Verification items for the finished model (mm, model axes). A direction names the side the tool comes from. Coordinates: 2 decimals unless noted, no trailing zeros. Order: outer loops, then holes, each group sorted by start corner. A loop starts at its lowest first (then second) coordinate and runs counter-clockwise, first axis right, second up. Notation, with made-up numbers: M 33,-2.75 L 77,-2.75 A20 ccw 77,1.25 Z; hole C -16.75,84.5 d1. An arc over 180 degrees is marked long. Return JSON: item names as keys, results as strings.
```python
from build123d import *

# Parameters (mm, degrees)
ESQUISSE1_W             = 170
ESQUISSE1_H             = 80
BOSS_EXTRU_1_DEPTH      = 3
ESQUISSE3_W             = 28
ESQUISSE3_H             = 3
ESQUISSE3_W_2           = 22
BOSS_EXTRU_2_DEPTH      = 3
ESQUISSE4_W             = 3
ESQUISSE4_H             = 19
ESQUISSE4_H_2           = 18
ESQUISSE4_H_3           = 19.233956883
BOSS_EXTRU_3_DEPTH      = 3
ESQUISSE5_W             = 3.071340823
ESQUISSE5_H             = 0.315544452
ENL_V_MAT_EXTRU_1_DEPTH = 3


with BuildPart() as part:
    # Esquisse1 → Boss.-Extru.1 (new body)
    with BuildSketch(Plane.XY):
        with Locations((40.41093995, 17.47440273)):
            Rectangle(ESQUISSE1_W, ESQUISSE1_H)
    extrude(amount=BOSS_EXTRU_1_DEPTH)

    # Esquisse3 → Boss.-Extru.2 (add)
    with BuildSketch(Plane(origin=(0, 0, 0), x_dir=(-1, 0, 0), z_dir=(0, 0, -1))):
        with Locations((-0.41093995, 58.97440273)):
            Rectangle(ESQUISSE3_W, ESQUISSE3_H)
        with Locations((-60.41093995, 58.97440273)):
            Rectangle(ESQUISSE3_W, ESQUISSE3_H)
        with Locations((-117.41093995, 58.97440273)):
            Rectangle(ESQUISSE3_W_2, ESQUISSE3_H)
        with Locations((-117.41093995, -24.02559727)):
            Rectangle(ESQUISSE3_W_2, ESQUISSE3_H)
        with Locations((-60.41093995, -24.02559727)):
            Rectangle(ESQUISSE3_W, ESQUISSE3_H)
        with Locations((-0.41093995, -24.02559727)):
            Rectangle(ESQUISSE3_W, ESQUISSE3_H)
    extrude(amount=-BOSS_EXTRU_2_DEPTH)

    # Esquisse4 → Boss.-Extru.3 (add)
    with BuildSketch(Plane.XY.offset(3)):
        with Locations((126.91093995, -13.02559727)):
            Rectangle(ESQUISSE4_W, ESQUISSE4_H)
        with Locations((126.91093995, 27.47440273)):
            Rectangle(ESQUISSE4_W, ESQUISSE4_H_2)
        with Locations((-46.08906005, 48.091381172)):
            Rectangle(ESQUISSE4_W, ESQUISSE4_H_3)
        with Locations((-46.08906005, 7.47440273)):
            Rectangle(ESQUISSE4_W, ESQUISSE4_H_2)
    extrude(amount=-BOSS_EXTRU_3_DEPTH)

    # Esquisse5 → Enlèv. mat.-Extru.1 (cut)
    with BuildSketch(Plane(origin=(0, 0, 0), x_dir=(-1, 0, 0), z_dir=(0, 0, -1))):
        with Locations((46.124730462, 57.632174956)):
            Rectangle(ESQUISSE5_W, ESQUISSE5_H)
    extrude(amount=-ENL_V_MAT_EXTRU_1_DEPTH, mode=Mode.SUBTRACT)


solid = part.part
```
Q1. Go/stop test with flat-tipped pins: pin 1 (1.5 mm diameter, centred on y = 59.5, z = 2, fed in from -X); pin 2 (1.5 mm diameter, centred on y = 47.5, z = 2, fed in from +X); pin 3 (1.5 mm diameter, centred on y = 26, z = 1.5, fed in from -X). Record where each tip stops, or that it passes through.
Values:
{"pin 1": "x = -13.59", "pin 2": "x = 125.41", "pin 3": "x = -44.59"}
Q2. Cross-section at A-A, the plane x = 32. Record the boundary of the cut face in (y, z), and give its area (3 significant figures).
Values:
{"outline": "M -22.53,0 L 57.47,0 L 57.47,3 L -22.53,3 Z", "area": "240 mm^2"}
Q3. Cross-section at B-B, the plane y = 30. Record the boundary of the cut face in (x, z), and give its area (3 significant figures).
Values:
{"outline": "M -44.59,0 L 128.41,0 L 128.41,3 L -44.59,3 Z", "area": "519 mm^2"}
Q4. Tool access check on faces 1 (the face through (125.411, 47, 1)), 2 (the face through (-30, 57.474, 1)), 3 (the face through (-46, 38.474, 2)), 4 (the face through (14.411, -24, 1)), 5 (the face through (106.411, 59, 1)). Record the directions out of +Z, -Z, +X, -X, +Y, -Y that give a thin tool (end or side, any length) a straight path to the whole face; none if there is none.
Values:
{"face 1": "+Z, -Z, +X", "face 2": "+Z, -Z, -X, +Y", "face 3": "+Z, -Z, -X", "face 4": "+Z, -Z, -Y", "face 5": "+Z, -Z, +Y"}
Q5. Material ranges on line 1 along X through (y, z) = (-9, 2.6); line 2 along Y through (x, z) = (77.5, 0.45); line 3 along X through (y, z) = (49.5, 1.85), recorded low to high.
Values:
{"line 1": "-44.59 to 128.41", "line 2": "-22.53 to 57.47", "line 3": "-47.59 to 125.41"}
